Geometry check sheet. Reference: the model listing, model coordinates, mm. Give positions to 0.01 mm unless a question says otherwise; leave off trailing zeros. Write each loop counter-clockwise with the first axis right and the second up, starting at its lowest first coordinate (ties: lowest second). Pieces come first, ordered by that corner, then holes. Notation, with made-up numbers: (61, 42) -> (86, 42) arc R20 cw to (86, 73) -> close; hole circle Ø7 at (-1, 6). An arc over 180 degrees is marked (long way). Write item = value, one per line. Start each with the question number.
1. Cross-section at A-A, the plane y = 1.4. Record the cut outline in (x, z).
2. Thickness scan on line 1 along Z through (x, y) = (-40, 3.3); line 2 along X through (y, z) = (1.6, -37.5). Record the ranges inside material, lowest first.
3. Depth check by flat-ended pin: P1, Ø7, axis at x = 40, z = 40, coming from the -Y side. Enter the tip coordinate at first touch or a pass-through.
```python
from build123d import *

# Parameters (mm, degrees)
SKETCH1_W                 = 100
SKETCH1_H                 = 100
BOSS_EXTRUDE1_DEPTH       = 5
F_8_0MM_DOWEL_HOLE1_D     = 8
F_8_0MM_DOWEL_HOLE1_DEPTH = 5
FILLET1_R                 = 10


with BuildPart() as part:
    # Sketch1 → Boss-Extrude1 (new body)
    with BuildSketch(Plane(origin=(0, 0, 0), x_dir=(1, 0, 0), z_dir=(0, 1, 0))):
        Rectangle(SKETCH1_W, SKETCH1_H)
    extrude(amount=BOSS_EXTRUDE1_DEPTH)

    # Ø8.0mm Dowel Hole1
    with Locations(Plane(origin=(0, 5, 0), x_dir=(1, 0, 0), z_dir=(0, 1, 0))):
        with Locations((-40, -40), (-40, 40), (40, 40), (40, -40)):
            Hole(F_8_0MM_DOWEL_HOLE1_D / 2, depth=F_8_0MM_DOWEL_HOLE1_DEPTH)

    # Fillet1
    fillet1_edges = [part.edges().sort_by_distance(p)[0] for p in [
        (-50, 2.5, -50),
        (50, 2.5, -50),
        (50, 2.5, 50),
        (-50, 2.5, 50),
    ]]
    fillet(fillet1_edges, radius=FILLET1_R)


solid = part.part
```
Answers:
q1.outline = (-50, -40) arc R10 ccw to (-40, -50) -> (40, -50) arc R10 ccw to (50, -40) -> (50, 40) arc R10 ccw to (40, 50) -> (-40, 50) arc R10 ccw to (-50, 40) -> close; hole circle Ø8 at (-40, -40); hole circle Ø8 at (-40, 40); hole circle Ø8 at (40, -40); hole circle Ø8 at (40, 40)
q2.line_1 = -50 to -44, -36 to 36, 44 to 50
q2.line_2 = -50 to -43.12, -36.88 to 36.88, 43.12 to 50
q3.P1 = through
